from build123d import *

# Parameters (mm, degrees)
F0_R     = 9.525
F1_DEPTH = 25.4
F3_DEPTH = 9.525
F5_W     = 10.315952
F5_H     = 10.315952
F6_DEPTH = 10.9728
F4_R     = 5.157976
F7_DEPTH = 25.401


with BuildPart() as f1:
    # F0 (on Front) → F1 (new body)
    with BuildSketch(Plane.XZ):
        Circle(F0_R)
    extrude(amount=F1_DEPTH)

    # F2 (on face) → F3 (cut)
    with BuildSketch(Plane.XZ.offset(25.4)):
        Polygon((6.310741, 3.674476), (-0.026819, 7.3025), (-6.33756, 3.628024), (-6.310741, -3.674476), (0.026819, -7.3025), (6.33756, -3.628024), align=None)
    extrude(amount=-F3_DEPTH, mode=Mode.SUBTRACT)

    # F5 (on Front) → F6 (cut)
    with BuildSketch(Plane.XZ):
        Rectangle(F5_W, F5_H)
    extrude(amount=F6_DEPTH, mode=Mode.SUBTRACT)

    # F4 (on face) → F7 (cut, through all)
    with BuildSketch(Plane(origin=(0, 0, 0), x_dir=(-1, 0, 0), z_dir=(0, 1, 0))):
        Circle(F4_R)
    extrude(amount=-F7_DEPTH, mode=Mode.SUBTRACT)


solid = f1.part
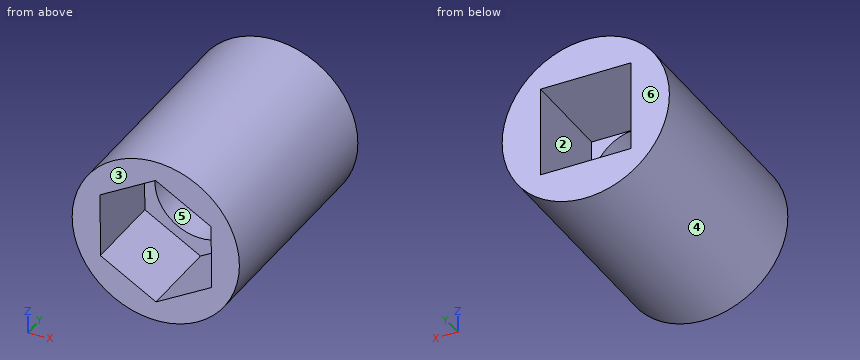
Build history of the part. All positions in model axes, mm. Face numbers are marked on the shaded views. A direction names the side the tool comes from. Coordinates: 2 decimals unless noted, no trailing zeros. Order: outer loops, then holes, each group sorted by start corner. A loop starts at its lowest first (then second) coordinate and runs counter-clockwise, first axis right, second up. Notation, with made-up numbers: (74.25, 68) -> (96.25, 68) arc R13 cw to (96.25, 75) -> close; hole circle Ø1 at (49.5, 30). An arc over 180 degrees is marked (long way). One line per item, written item: value.
(1) Drop flat-ended pins along their axis: pin 1 Ø1.5 at (x, z) = (-3, 2.5) entering from +Y; pin 2 Ø1.5 at (x, y) = (5.5, -15) entering from +Z; pin 3 Ø1 at (x, z) = (2, -4.5) entering from -Y (3 decimals); pin 4 Ø1.5 at (y, z) = (-7.5, -2.5) entering from +X. Give the stop position or say it passes through.
Checked values:
pin 1: through
pin 2: z = 8.26
pin 3: y = -15.875
pin 4: x = 9.36
(2) Tool access for the marked faces 1, 2 and 3: list every direction of +Z, -Z, +X, -X, +Y, -Y with a clear straight run to the whole face (end or side of a thin tool).
Checked values:
face 1: -Y
face 2: +Y
face 3: +Z, -Z, +X, -X, -Y
(3) Mould opens along X. For the marked faces 4, 5 and 6 say: pulls with the +X half, pulls with the -X half, needs draft (parallel to the pull), parting line crosses it, or undercut.
Checked values:
face 4: parting line crosses it
face 5: undercut
face 6: needs draft
(4) Probe line 1 (Z direction, x = 0, y = -13.65) (3 decimals); line 2 (X direction, y = -10.25, z = -2); line 3 (Z direction, x = 4.5, y = -7). List the from-to ranges inside material, lowest first. Write a range as [from, to].
Checked values:
line 1: [-9.525, -5.158], [5.158, 9.525]
line 2: [-9.31, -5.16], [5.16, 9.31]
line 3: [-8.39, -5.16], [5.16, 8.39]
(5) Slice it at B-B, the plane z = -2.25. List the corners of the cut face in (x, y) (1 decimal), plus the area to 3 significant figures.
Checked values:
outline: (-9.3, -25.4) -> (-6.3, -25.4) -> (-6.3, -15.9) -> (-4.6, -15.9) -> (-4.6, -11) -> (-5.2, -11) -> (-5.2, 0) -> (-9.3, 0) -> close; (4.6, -15.9) -> (6.3, -15.9) -> (6.3, -25.4) -> (9.3, -25.4) -> (9.3, 0) -> (5.2, 0) -> (5.2, -11) -> (4.6, -11) -> close
area: 191 mm2
(6) Slice it at C-C, the plane x = 1.75. List the corners of the cut face in (y, z) (3 decimals), plus the area to 3 significant figures.
Checked values:
outline: (-25.4, -9.363) -> (0, -9.363) -> (0, -5.158) -> (-10.973, -5.158) -> (-10.973, -4.852) -> (-15.875, -4.852) -> (-15.875, -6.299) -> (-25.4, -6.299) -> close; (-25.4, 6.285) -> (-15.875, 6.285) -> (-15.875, 4.852) -> (-10.973, 4.852) -> (-10.973, 5.158) -> (0, 5.158) -> (0, 9.363) -> (-25.4, 9.363) -> close
area: 195 mm2
(7) Slice it at D-D, the plane z = 7. List the corners of the cut face in (x, y) (3 decimals).
Checked values:
outline: (-6.46, -25.4) -> (-0.546, -25.4) -> (-0.546, -15.875) -> (0.502, -15.875) -> (0.502, -25.4) -> (6.46, -25.4) -> (6.46, 0) -> (-6.46, 0) -> close
